```python
from build123d import *

# Parameters (mm, degrees)
BOX047_W               = 26
BOX047_H               = 132
BOX047_DEPTH           = 20
BOX047_PLACEMENT_ANGLE = 135
BOX046_W               = 190
BOX046_H               = 158
BOX046_DEPTH           = 20
BOX046_PLACEMENT_ANGLE = 315


with BuildPart() as cube009:
    # Box047 → Box047 (new body)
    with BuildSketch(Plane.XY):
        with Locations((13, 66)):
            Rectangle(BOX047_W, BOX047_H)
    extrude(amount=BOX047_DEPTH)


with BuildPart() as cube009_1:
    # Box047 placement: moved
    add(cube009.part.moved(Location((50.558135, -94.102291, 40.5))).rotate(Axis((50.558135, -94.102291, 40.5), (0, 0, -1)), BOX047_PLACEMENT_ANGLE))


with BuildPart() as fusion012:
    # Box046 → Box046 (new body)
    with BuildSketch(Plane.XY):
        with Locations((95, 79)):
            Rectangle(BOX046_W, BOX046_H)
    extrude(amount=BOX046_DEPTH)


with BuildPart() as fusion012_1:
    # Box046 placement: moved
    add(fusion012.part.moved(Location((32.880465, -76.424621, 40.5))).rotate(Axis((32.880465, -76.424621, 40.5), (0, 0, 1)), BOX046_PLACEMENT_ANGLE))

    # Fusion012: union Cube009
    add(cube009_1.part)


solid = fusion012_1.part
```
Geometry check sheet. Reference: the model listing, model coordinates, mm. A direction names the side the tool comes from. Give positions to 0.01 mm unless a question says otherwise; leave off trailing zeros. Order: outer loops, then holes, each group sorted by start corner. A loop starts at its lowest first (then second) coordinate and runs counter-clockwise, first axis right, second up.
1. Section check B-B, the plane y = -56. Enter the section's corners in (x, z).
2. Gauge pin test, flat ends, axial feed: pin 1 Ø3 at (y, z) = (-177, 57) entering from -X; pin 2 Ø4 at (y, z) = (-109.5, 55) entering from -X; pin 3 Ø2 at (x, z) = (131.5, 51) entering from +Y. Record the tip position at first contact, or that the pin passes through.
3. Section check C-C, the plane x = 162.5. Enter the section's corners in (y, z), and give its area (3 significant figures).
4. Release check for a two-part mould opening along Y. For faces 1 (the face through (147, -95, 40.5)), 2 (the face through (78.189, -158.503, 50.36)), 3 (the face through (41.596, -85.14, 50.36)), 4 (the face through (41.49, -103.17, 50.36)) record: pulls with the +Y half, pulls with the -Y half, needs draft (parallel to the pull), parting line crosses it, or undercut.
5. Section check A-A, the plane z = 43.75. Enter the section's corners in (x, y), and give its area (3 significant figures).
6. Thickness scan on L1, parallel to X at y = -198, z = 44; L2, parallel to X at y = -201, z = 52.25; L3, parallel to Y at x = 49, z = 59.25. Record the ranges inside material, lowest first.
7. Access from +Z, -Z, +X, -X, +Y, -Y to the whole of each face (thin tool, end or side, straight path). Record for faces 5 (the face through (87.96, -21.345, 50.36)), 6 (the face through (134.833, -196.504, 50.36)).
Values follow:
1. outline: (53.31, 40.5) - (235.9, 40.5) - (235.9, 60.5) - (53.31, 60.5) - close
2. pin 1: stops at x = 95.19
2. pin 2: stops at x = 33.16
2. pin 3: stops at y = 23.19
3. outline: (-206.04, 40.5) - (17.4, 40.5) - (17.4, 60.5) - (-206.04, 60.5) - close
3. area: 4,470 mm2
4. face 1: needs draft
4. face 2: pulls with the -Y half
4. face 3: undercut
4. face 4: undercut
5. outline: (32.17, -112.49) - (125.51, -205.83) - (143.9, -187.44) - (167.23, -210.77) - (278.95, -99.05) - (144.6, 35.3) - (32.88, -76.42) - (50.56, -94.1) - close
5. area: 33,500 mm2
6. L1: x = 117.69 to 133.34, 154.46 to 180.01
6. L2: x = 120.69 to 130.34, 157.46 to 177.01
6. L3: y = -129.31 to -95.66, -92.54 to -60.31
7. face 5: +Z, -Z, -X, +Y
7. face 6: +Z, -Z, -Y
